Part model, mm, in its own coordinate system. Face numbers are marked on the shaded views. Give positions to 0.01 mm unless a question says otherwise; leave off trailing zeros. Order: outer loops, then holes, each group sorted by start corner. A loop starts at its lowest first (then second) coordinate and runs counter-clockwise, first axis right, second up. Notation, with made-up numbers: (57.25, -28) - (69.25, -28) arc R34 cw to (69.25, 7) - close; hole circle Ø1 at (55, -28.75). An arc over 180 degrees is marked (long way). Use one line per item in the form item = value. Start each with the question number.
1. Pull direction Y, two halves, no side cores. Call the marked faces 1, 2, 3 and 4: +Y half, -Y half, draft (parallel to the pull), parting line (faces both ways), or undercut.
2. Band-saw the part on A-A, the plane x = 3. List the corners of the cut face in (y, z).
3. Pin check, flat tips, straight feed: P1, Ø4, axis at x = 9.5, z = 3, coming from the +Y side; P2, Ø5, axis at x = 11.5, y = 0.5, coming from the +Z side; P3, Ø1.5, axis at x = 3, z = 1.5, coming from the +Y side; P4, Ø6, axis at y = 3, z = 0.5, coming from the -X side. Stop position of each tip, or through.
4. Drill centre lines: line 1 (X direction, y = -4, z = 2); line 2 (X direction, y = -2.25, z = 0.5); line 3 (Y direction, x = 1.75, z = 3). Where is each one in solid material? Low to high.
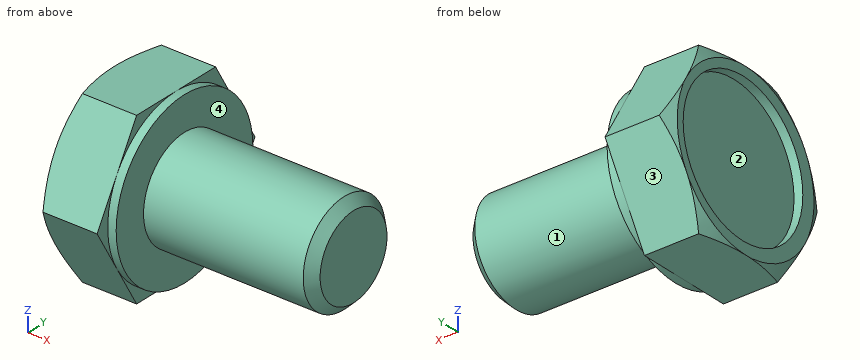
from build123d import *

# Parameters (mm, degrees)
BASEHEAD_DEPTH     = 4.15
INDENT_START       = -0.51875
INDENT_2_OUTLINE_R = 4.375
INDENT_2_DEPTH     = 0.51875
SKETCH4_W          = 0.5
SKETCH4_H          = 10.773502692


# Read off the part's stored shape, not the designer's step: Indent
with BuildPart() as part:
    # Sketch1 → BaseHead (new body)
    with BuildSketch(Plane(origin=(0, 0, 0), x_dir=(0, 0, -1), z_dir=(1, 0, 0))):
        Polygon((5, 2.886751346), (5, -2.886751346), (0, -5.773502692), (-5, -2.886751346), (-5, 2.886751346), (0, 5.773502692), align=None)
    extrude(amount=BASEHEAD_DEPTH)

    # Indent outline → Indent (revolve)
    with BuildSketch(Plane.YX):
        Polygon((3, 4.15), (3, 13.5955), (2.4455, 14.15), (0, 14.15), (0, 4.15), align=None)
    revolve(axis=Axis((0, 0, 0), (1, 0, 0)))

    # Indent 2 outline → Indent 2 (cut)
    with BuildSketch(Plane.ZY.offset(INDENT_START)):
        with Locations((0.033212245, 0.192376607)):
            Circle(INDENT_2_OUTLINE_R)
    extrude(amount=INDENT_2_DEPTH, mode=Mode.SUBTRACT)

    # Sketch3 → HeadChamfer (revolve, cut)
    with BuildSketch(Plane.XY, mode=Mode.PRIVATE) as headchamfer_sk:
        Polygon((0, 5), (3.333333333, 10.773502692), (3.333333333, 15.773502692), (-10, 15.773502692), (-10, 5), align=None)
    revolve(headchamfer_sk.sketch.rotate(Axis((0, 0, 0), (1, 0, 0)), 90), axis=Axis((0, 0, 0), (1, 0, 0)), mode=Mode.SUBTRACT)

    # Sketch4 → BearingFace (revolve, cut)
    with BuildSketch(Plane.XY, mode=Mode.PRIVATE) as bearingface_sk:
        with Locations((3.9, 10.386751346)):
            Rectangle(SKETCH4_W, SKETCH4_H)
    revolve(bearingface_sk.sketch.rotate(Axis((0, 0, 0), (1, 0, 0)), 90), axis=Axis((0, 0, 0), (1, 0, 0)), mode=Mode.SUBTRACT)


solid = part.part
From the geometry:
q1.face_1 = parting line
q1.face_2 = undercut
q1.face_3 = +Y half
q1.face_4 = draft
q2.outline = (-5.77, 0) - (-2.89, -5) - (2.89, -5) - (5.77, 0) - (2.89, 5) - (-2.89, 5) - close
q3.P1 = 2.83
q3.P2 = 3
q3.P3 = 5.34
q3.P4 = 0
q4.line_1 = 0 to 4.15
q4.line_2 = 0.52 to 14.15
q4.line_3 = -4.04 to 4.04
